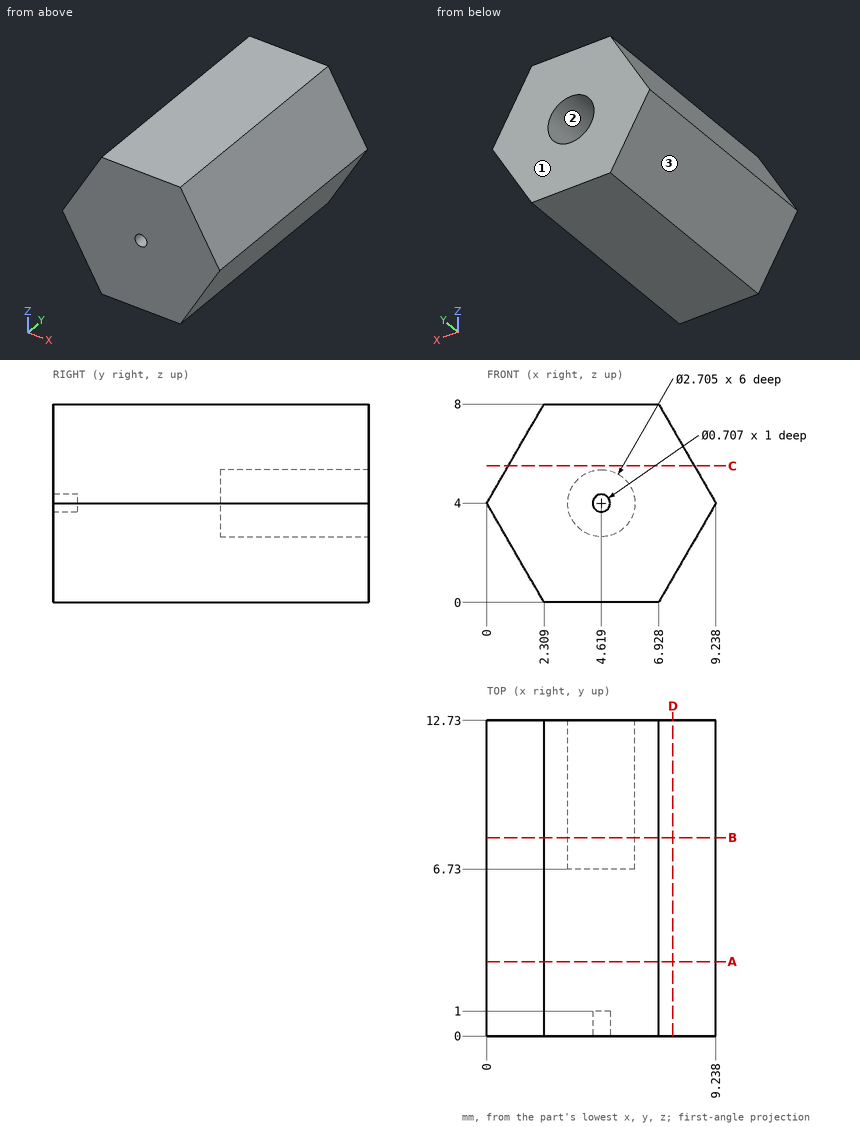
Input: dimensioned drawing with shaded views. Units: mm. Origin: part minimum x, y, z. Give positions to 0.01 mm unless a question says otherwise; leave off trailing zeros. Write each loop counter-clockwise with the first axis right and the second up, starting at its lowest first coordinate (ties: lowest second). Pieces come first, ordered by that corner, then holes. Notation, with made-up numbers: (16, -28) -> (44, -28) arc R21 ccw to (44, 9) -> close; hole circle Ø8 at (22, 39). An arc over 180 degrees is marked (long way). Return JSON: item names as keys, results as strings. Group by question number.
1. Mould query, pull axis Z, two halves, no side actions, for the marked faces 1, 2 and 3. Classes: +Z half, -Z half, draft (parallel to the pull), parting line (faces both ways), or undercut.
2. Section D-D, the plane x = 7.5. Output: boundary loops of the cut face in (y, z).
3. Section C-C, the plane z = 5.5. Output: boundary loops of the cut face in (x, y).
4. Material intervals for line 1 (Y direction, x = 5, z = 4.75); line 2 (Z direction, x = 3.75, y = 11) (1 decimal); line 3 (X direction, y = 2.5, z = 3), sorted ascending. Write a range as from..to.
5. Section A-A, the plane y = 3. Output: boundary loops of the cut face in (x, z).
6. Pin query (flat end, axial travel): pin 1 Ø4 at (x, y) = (1.5, 1.5) entering from -Z; pin 2 Ø1 at (y, z) = (11, 2.5) entering from -X; pin 3 Ø1.5 at (y, z) = (7.5, 1.5) entering from -X; pin 4 Ø0.8 at (x, z) = (5, 3.5) entering from +Y. Return the tip coordinate at first contact, or that it passes through.
7. Section B-B, the plane y = 8. Output: boundary loops of the cut face in (x, z) (1 decimal).
Determined:
{
 "1": {"face 1": "draft", "face 2": "undercut", "face 3": "-Z half"},
 "2": {"outline": "(0, 0.99) -> (12.73, 0.99) -> (12.73, 7.01) -> (0, 7.01) -> close"},
 "3": {"outline": "(0.87, 0) -> (8.37, 0) -> (8.37, 12.73) -> (0.87, 12.73) -> close"},
 "4": {"line 1": "y = 0..6.73", "line 2": "z = 0..3, 5..8", "line 3": "x = 0.58..8.66"},
 "5": {"outline": "(0, 4) -> (2.31, 0) -> (6.93, 0) -> (9.24, 4) -> (6.93, 8) -> (2.31, 8) -> close"},
 "6": {"pin 1": "stops at z = 0", "pin 2": "stops at x = 0.58", "pin 3": "stops at x = 1.01", "pin 4": "stops at y = 6.73"},
 "7": {"outline": "(0, 4) -> (2.3, 0) -> (6.9, 0) -> (9.2, 4) -> (6.9, 8) -> (2.3, 8) -> close; hole circle Ø2.7 at (4.6, 4)"}
}
